from build123d import *

# Parameters (mm, degrees)
SKETCH1_W               = 30
SKETCH1_H               = 93
BOSS_EXTRUDE1_DEPTH     = 8
SKETCH2_W               = 10
SKETCH2_H               = 12
CUT_EXTRUDE1_DEPTH      = 8
SKETCH3_R               = 2.25
CUT_EXTRUDE2_DEPTH      = 56.91287866
FILLET1_R               = 2
CUT_EXTRUDE3_DEPTH      = 50.51009998
FILLET2_R               = 3
CUT_EXTRUDE4_DEPTH      = 50.51009998
CUT_EXTRUDE4_DEPTH_BACK = 50.51009998
FILLET3_R               = 1
FILLET4_R               = 0.5
SKETCH8_W               = 20
SKETCH8_H               = 8
BOSS_EXTRUDE2_DEPTH     = 5
CUT_EXTRUDE5_DEPTH      = 59.747340518
CUT_EXTRUDE5_DEPTH_BACK = 5
SKETCH9_R               = 1.502727392
CHAMFER1_SIZE           = 4
FILLET5_R               = 1


with BuildPart() as part:
    # Sketch1 → Boss-Extrude1 (new body)
    with BuildSketch(Plane(origin=(0, 0, 0), x_dir=(1, 0, 0), z_dir=(0, 1, 0))):
        Rectangle(SKETCH1_W, SKETCH1_H)
    extrude(amount=BOSS_EXTRUDE1_DEPTH)

    # Sketch2 → Cut-Extrude1 (cut)
    with BuildSketch(Plane(origin=(0, 8, 0), x_dir=(1, 0, 0), z_dir=(0, 1, 0))):
        with Locations((0, -40.5)):
            Rectangle(SKETCH2_W, SKETCH2_H)
    extrude(amount=-CUT_EXTRUDE1_DEPTH, mode=Mode.SUBTRACT)

    # Sketch3 → Cut-Extrude2 (cut, through all)
    with BuildSketch(Plane(origin=(15, 0, 0), x_dir=(0, 0, -1), z_dir=(1, 0, 0))):
        with Locations((-41.5, 4)):
            Circle(SKETCH3_R)
    extrude(amount=-CUT_EXTRUDE2_DEPTH, mode=Mode.SUBTRACT)

    # Fillet1
    fillet1_edges = [part.edges().sort_by_distance(p)[0] for p in [
        (10, 0, 46.5),
        (-10, 8, 46.5),
        (10, 8, 46.5),
        (-10, 0, 46.5),
        (0, 0, -46.5),
        (0, 8, -46.5),
    ]]
    fillet(fillet1_edges, radius=FILLET1_R)

    # Sketch4 → Cut-Extrude3 (cut, through all)
    with BuildSketch(Plane(origin=(0, 8, 0), x_dir=(1, 0, 0), z_dir=(0, 1, 0))):
        Polygon((5, 26), (-10, 26), (1.715328467, 14.284671533), align=None)
        Polygon((10, 6), (10, 26), (5.620437956, 10.379562044), align=None)
        Polygon((-10, -7.5), (-10, -27.5), (-5.620437956, -11.879562044), align=None)
        Polygon((-5, -27.5), (10, -27.5), (-1.715328467, -15.784671533), align=None)
        Polygon((-10, 18.928932188), (-10, -0.428932188), (-4.072028946, -6.356903242), (0.166919457, 8.762012731), align=None)
        Polygon((9.732575479, -20.161507667), (9.732575479, -0.803643291), (4.072028946, 4.856903242), (-0.166919457, -10.262012731), align=None)
    extrude(amount=-CUT_EXTRUDE3_DEPTH, mode=Mode.SUBTRACT)

    # Fillet2
    fillet2_edges = [part.edges().sort_by_distance(p)[0] for p in [
        (0, 0, 34.5),
    ]]
    fillet(fillet2_edges, radius=FILLET2_R)

    # Sketch6 → Cut-Extrude4 (cut, two sides: drawn at the far end of the back side and taken through both)
    with BuildSketch(Plane(origin=(0, 8, 0), x_dir=(1, 0, 0), z_dir=(0, 1, 0)).offset(-CUT_EXTRUDE4_DEPTH_BACK)):
        with BuildLine():
            Line((-7.477541934, 46.5), (-15, 46.5))
            Line((-15, 46.5), (-15, 19.983197599))
            ThreePointArc((-15, 19.983197599), (-9.022671438, 32.612921347), (-7.477541934, 46.5))
        make_face()
        with BuildLine():
            Line((15, 46.5), (15, 19.983197599))
            ThreePointArc((15, 19.983197599), (9.022671438, 32.612921347), (7.477541934, 46.5))
            Line((7.477541934, 46.5), (15, 46.5))
        make_face()
    extrude(amount=CUT_EXTRUDE4_DEPTH + CUT_EXTRUDE4_DEPTH_BACK, mode=Mode.SUBTRACT)

    # Sketch5 → Cut-Revolve1 (revolve, cut)
    with BuildSketch(Plane(origin=(0, 0, 0), x_dir=(0, 0, -1), z_dir=(1, 0, 0))):
        with BuildLine():
            Line((38.5, 8), (38.5, 0))
            Line((38.5, 0), (42, 0))
            ThreePointArc((42, 0), (43.815072906, 4), (42, 8))
            Line((42, 8), (38.5, 8))
        make_face()
    revolve(axis=Axis((0, 8, -38.5), (0, -1, 0)), mode=Mode.SUBTRACT)

    # Fillet3
    fillet3_edges = [part.edges().sort_by_distance(p)[0] for p in [
        (0, 8, -35),
        (0, 0, -35),
    ]]
    fillet(fillet3_edges, radius=FILLET3_R)

    # Fillet4
    fillet4_edges = [part.edges().sort_by_distance(p)[0] for p in [
        (-10, 4, -18.928932188),
        (0.166919457, 4, -8.762012731),
        (-4.072028946, 4, 6.356903242),
        (-10, 4, 0.428932188),
        (-1.715328467, 4, 15.784671533),
        (10, 4, 27.5),
        (-5, 4, 27.5),
        (10, 4, -6),
        (5.620437956, 4, -10.379562044),
        (10, 4, -26),
        (-5.620437956, 4, 11.879562044),
        (-10, 4, 27.5),
        (9.732575479, 4, 20.161507667),
        (-0.166919457, 4, 10.262012731),
        (4.072028946, 4, -4.856903242),
        (9.732575479, 4, 0.803643291),
        (5, 4, -26),
        (1.715328467, 4, -14.284671533),
        (-10, 4, -26),
    ]]
    fillet(fillet4_edges, radius=FILLET4_R)

    # Sketch8 → Boss-Extrude2 (add)
    with BuildSketch(Plane(origin=(15, 0, 0), x_dir=(0, 0, -1), z_dir=(1, 0, 0))):
        with Locations((-0.5, 4)):
            Rectangle(SKETCH8_W, SKETCH8_H)
    extrude(amount=BOSS_EXTRUDE2_DEPTH)

    # Sketch9 → Cut-Extrude5 (cut, two sides: drawn at the far end of the back side and taken through both)
    with BuildSketch(Plane(origin=(20, 0, 0), x_dir=(0, 0, -1), z_dir=(1, 0, 0)).offset(-CUT_EXTRUDE5_DEPTH_BACK)):
        with Locations((4, 4)):
            Circle(SKETCH9_R)
    extrude(amount=CUT_EXTRUDE5_DEPTH + CUT_EXTRUDE5_DEPTH_BACK, mode=Mode.SUBTRACT)

    # Chamfer1
    chamfer1_edges = [part.edges().sort_by_distance(p)[0] for p in [
        (15, 4, 10.5),
        (15, 4, -9.5),
    ]]
    chamfer(chamfer1_edges, length=CHAMFER1_SIZE)

    # Fillet5
    fillet5_edges = [part.edges().sort_by_distance(p)[0] for p in [
        (20, 4, 10.5),
        (15, 4, 14.5),
        (15, 4, -19.983197599),
        (20, 4, -9.5),
    ]]
    fillet(fillet5_edges, radius=FILLET5_R - 0.0001)  # a hair under: the kernel refuses the full size


solid = part.part
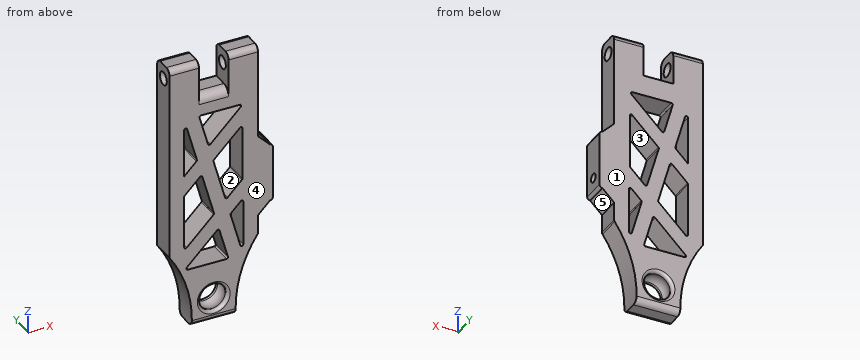
Verification items for the finished model (mm, model axes). Face numbers are marked on the shaded views. A direction names the side the tool comes from. Coordinates: 2 decimals unless noted, no trailing zeros. Write each loop counter-clockwise with the first axis right and the second up, starting at its lowest first coordinate (ties: lowest second). Pieces come first, ordered by that corner, then holes. Notation, with made-up numbers: (73, 10) - (82, 10) arc R18 cw to (82, 17) - close; hole circle Ø11 at (2, 42). An arc over 180 degrees is marked (long way). Answer as a JSON object with one key per item and string values.
(1) Tool access check on the marked faces 1 and 2. Record the directions out of +Z, -Z, +X, -X, +Y, -Y that give a thin tool (end or side, any length) a straight path to the whole face; none if there is none.
Report:
{"face 1": "+Z, -Z, +X, -X, +Y", "face 2": "+Y, -Y"}
(2) Cross-section at C-C on z = 23. Record the cut outline in (x, y), plus the area to 3 significant figures.
Report:
{"outline": "(-15, 0) - (-10, 0) - (-10, 8) - (-15, 8) - close; (-8.74, 0) - (-3.74, 0) - (-3.74, 8) - (-8.74, 8) - close; (5.5, 0) - (15, 0) - (15, 8) - (5.5, 8) - close", "area": "156 mm^2"}
(3) Cross-section at D-D on z = -31. Record the cut outline in (x, y), plus the area to 3 significant figures.
Report:
{"outline": "(-9.52, 0) - (9.52, 0) - (9.52, 8) - (-9.52, 8) - close", "area": "152 mm^2"}
(4) Cross-section at A-A on z = 35.5. Record the cut outline in (x, y), plus the area to 3 significant figures.
Report:
{"outline": "(-15, 0) - (-5, 0) - (-5, 8) - (-15, 8) - close; (5, 0) - (15, 0) - (15, 8) - (5, 8) - close", "area": "160 mm^2"}
(5) Mould release check, pull along Z, two halves, no side actions. Record for the marked faces 3, 4 and 5: pulls with the +Z half, pulls with the -Z half, needs draft (parallel to the pull), parting line crosses it, or undercut.
Report:
{"face 3": "undercut", "face 4": "needs draft", "face 5": "pulls with the -Z half"}
(6) Thickness scan on line 1 along Y through (x, z) = (7, 41.5); line 2 along X through (y, z) = (2, 4.5); line 3 along X through (y, z) = (0.75, -22.5). Record the ranges inside material, lowest first.
Report:
{"line 1": "0 to 1.75, 6.25 to 8", "line 2": "-15 to -5.93, -3.55 to 1.45, 9.73 to 20", "line 3": "-13.38 to -6.5, 4.02 to 9.02, 9.98 to 13.38"}
(7) Gauge pin test, flat ends, axial feed: pin 1 Ø4 at (y, z) = (4.5, 14.5) entering from +X; pin 2 Ø1.5 at (y, z) = (4.5, -4.5) entering from +X; pin 3 Ø4 at (x, y) = (-2.5, 5.5) entering from +Z. Record the tip position at first contact, or that the pin passes through.
Report:
{"pin 1": "x = 17", "pin 2": "x = 15", "pin 3": "z = 34.5"}
(8) Cross-section at B-B on y = 4. Give the number of separate pieces and of enclosed holes in the cut face, plus the area to 3 significant figures.
Report:
{"separate pieces": "3", "enclosed holes": "7", "area": "1,740 mm^2"}
